from build123d import *

# Parameters (mm, degrees)
F0_W      = 36
F0_H      = 15
F1_DEPTH  = 4
F2_R      = 7.5
F3_DEPTH  = 6
F4_R      = 7.49999
F6_DEPTH  = 8
F7_R      = 1.725
F8_DEPTH  = 4
F7_R_2    = 3.5
F9_DEPTH  = 1
F10_R     = 3.125
F11_DEPTH = 2
F12_R     = 3.2
F13_DEPTH = 0.1
F14_R     = 7
F15_DEPTH = 2.6
F17_DEPTH = 0.2


# Not quite as in the source:
# - a fillet or chamfer is up to 0.001 mm smaller than in the source, because OpenCascade refuses the exact size


with BuildPart() as f1:
    # F0 (on Top) → F1 (new body)
    with BuildSketch(Plane.XY):
        Rectangle(F0_W, F0_H)
    extrude(amount=F1_DEPTH)

    # F2 (on face) → F3 (join)
    with BuildSketch(Plane.XY.offset(4)):
        Circle(F2_R)
    extrude(amount=F3_DEPTH)

    # F4 (radius 7.5 in the source; OpenCascade refuses exactly that, so slightly less here)
    f4_edges = [f1.edges().sort_by_distance(p)[0] for p in [
        (-18, -7.5, 2),
        (-18, 7.5, 2),
        (18, -7.5, 2),
        (18, 7.5, 2),
    ]]
    fillet(f4_edges, radius=F4_R)

    # F5 (on face) → F6 (cut)
    with BuildSketch(Plane(origin=(0, 0, 0), x_dir=(1, 0, 0), z_dir=(0, 0, -1))):
        Polygon((2.8867513459, 5), (-2.8867513459, 5), (-5.7735026919, 0), (-2.8867513459, -5), (2.8867513459, -5), (5.7735026919, 0), align=None)
    extrude(amount=-F6_DEPTH, mode=Mode.SUBTRACT)

    # F7 (on face) → F8 (cut, through all)
    with BuildSketch(Plane.XY.offset(4)):
        with Locations((12, 0)):
            Circle(F7_R)
        with Locations((-12, 0)):
            Circle(F7_R)
    extrude(amount=-F8_DEPTH, mode=Mode.SUBTRACT)

    # F7 (on face) → F9 (cut)
    with BuildSketch(Plane.XY.offset(4)):
        with Locations((-12, 0)):
            Circle(F7_R_2)
        with Locations((-12, 0)):
            Circle(F7_R, mode=Mode.SUBTRACT)
        with Locations((12, 0)):
            Circle(F7_R_2)
        with Locations((12, 0)):
            Circle(F7_R, mode=Mode.SUBTRACT)
    extrude(amount=-F9_DEPTH, mode=Mode.SUBTRACT)

    # F10 (on face) → F11 (cut, through all)
    with BuildSketch(Plane.XY.offset(10)):
        Circle(F10_R)
    extrude(amount=-F11_DEPTH, mode=Mode.SUBTRACT)

    # F12 (on face) → F13 (join)
    with BuildSketch(Plane(origin=(0, 0, 8), x_dir=(1, 0, 0), z_dir=(0, 0, -1))):
        Circle(F12_R)
    extrude(amount=-F13_DEPTH)

    # F14 (on face) → F15 (cut)
    with BuildSketch(Plane(origin=(0, 0, 0), x_dir=(1, 0, 0), z_dir=(0, 0, -1))):
        Circle(F14_R)
    extrude(amount=-F15_DEPTH, mode=Mode.SUBTRACT)

    # F16 (on face) → F17 (join)
    with BuildSketch(Plane(origin=(0, 0, 2.6), x_dir=(1, 0, 0), z_dir=(0, 0, -1))):
        Polygon((2.8867513459, 5), (-2.8867513459, 5), (-5.7735026919, 0), (-2.8867513459, -5), (2.8867513459, -5), (5.7735026919, 0), align=None)
    extrude(amount=-F17_DEPTH)


solid = f1.part
Geometry check sheet. Reference: the model listing, model coordinates, mm. A direction names the side the tool comes from. Round coordinates to 2 decimals unless told otherwise and drop trailing zeros. Order: outer loops, then holes, each group sorted by start corner. A loop starts at its lowest first (then second) coordinate and runs counter-clockwise, first axis right, second up. Notation, with made-up numbers: M -35.5,30.5 L -9.5,30.5 A23 ccw -9.5,47.5 Z; hole C 76,38.25 d9. An arc over 180 degrees is marked long. Answer in a Markdown table with one row per item. Add a question column.
Item 1: Sectioned sample at C-C, the plane z = 2. State how many separate pieces and enclosed holes the cut face has, plus the area to 3 significant figures.
Item 2: Sectioned sample at A-A, the plane z = 7.25. Enter the section's corners in (x, y).
Item 3: Depth check by flat-ended pin: pin 1 Ø4 at (x, y) = (0, 0) entering from -Z; pin 2 Ø1.5 at (x, z) = (-6.5, 6) entering from +Y; pin 3 Ø1 at (y, z) = (5, 5.5) entering from +X; pin 4 Ø3 at (x, y) = (12, 0) entering from +Z. Enter the tip coordinate at first touch or a pass-through.
Item 4: Sectioned sample at B-B, the plane x = 12. Enter the section's corners in (y, z) (3 decimals), plus the area to 3 significant figures.
Item 5: Material ranges on L1, parallel to Z at x = -3, y = -2.5; L2, parallel to Y at x = 0, z = 9 (3 decimals); L3, parallel to X at y = 0.25, z = 1.25, recorded low to high. Write a range as [from, to].
Item 6: Draft check along Y on faces 1 (the face through (-11, 2, 3)), 2 (the face through (-15.745, -5.361, 2.028)), 3 (the face through (-15.745, 5.361, 2.028)). Enter one of: released by +Y, released by -Y, zero draft, split by the parting line, or undercut.
Item 7: Sectioned sample at D-D, the plane y = -6.5. Enter the section's corners in (x, z), plus the area to 3 significant figures.
Item 8: Set-up check for faces 4 (the face through (0, -7.5, 2)), 5 (the face through (4.31, 2.535, 5.364)), 6 (the face through (2.98, 0.94, 9.06)): record each of +Z, -Z, +X, -X, +Y, -Y from which the full face is reachable in a straight line by a thin tool's end or side.
Filled in:
| question | item | result |
|---|---|---|
| 1 | separate pieces | 1 |
| 1 | enclosed holes | 3 |
| 1 | area | 319 mm² |
| 2 | outline | C 0,0 d15; hole M -5.77,0 L -2.89,-5 L 2.89,-5 L 5.77,0 L 2.89,5 L -2.89,5 Z |
| 3 | pin 1 | stops at z = 2.6 |
| 3 | pin 2 | stops at y = 4.82 |
| 3 | pin 3 | stops at x = 6 |
| 3 | pin 4 | passes through |
| 4 | outline | M -7.348,0 L -1.725,0 L -1.725,3 L -3.5,3 L -3.5,4 L -7.348,4 Z; M 1.725,0 L 7.348,0 L 7.348,4 L 3.5,4 L 3.5,3 L 1.725,3 Z |
| 4 | area | 41.4 mm² |
| 5 | L1 | z = [2.6, 2.8], [8, 10] |
| 5 | L2 | y = [-7.5, -3.125], [3.125, 7.5] |
| 5 | L3 | x = [-18, -13.71], [-10.29, -7], [7, 10.29], [13.71, 18] |
| 6 | face 1 | undercut |
| 6 | face 2 | released by -Y |
| 6 | face 3 | released by +Y |
| 7 | outline | M -14.24,0 L -2.6,0 L -2.6,2.6 L 2.6,2.6 L 2.6,0 L 14.24,0 L 14.24,4 L 3.74,4 L 3.74,10 L -3.74,10 L -3.74,4 L -14.24,4 Z |
| 7 | area | 145 mm² |
| 8 | face 4 | +Z, -Z, +X, -X, -Y |
| 8 | face 5 | none |
| 8 | face 6 | +Z |
